Input: part model. Units: mm. Frame: model coordinates. Give positions to 0.01 mm unless a question says otherwise; leave off trailing zeros. Loops run counter-clockwise (first coordinate to the right, second up) from the corner with the lowest first, then second, coordinate; pieces in that order, holes last.
from build123d import *

# Parameters (mm, degrees)
SKETCH1_W          = 600
SKETCH1_H          = 600
PLATE_DEPTH        = 20
SKETCH2_R          = 87.5
BEARING_HOLE_DEPTH = 18
SKETCH3_R          = 84.25
CUT_EXTRUDE2_DEPTH = 18
SKETCH4_W          = 555
SKETCH4_H          = 555
SKETCH4_W_2        = 550
SKETCH4_H_2        = 550
CUT_EXTRUDE3_DEPTH = 10


with BuildPart() as part:
    # Sketch1 → plate (new body)
    with BuildSketch(Plane(origin=(0, 0, 0), x_dir=(1, 0, 0), z_dir=(0, 1, 0))):
        Rectangle(SKETCH1_W, SKETCH1_H)
    extrude(amount=PLATE_DEPTH)

    # Sketch2 → bearing-hole (cut)
    with BuildSketch(Plane(origin=(0, 20, 0), x_dir=(1, 0, 0), z_dir=(0, 1, 0))):
        with Locations(Location((0, 0, 0), (0, 0, 270))):
            Circle(SKETCH2_R)
    extrude(amount=-BEARING_HOLE_DEPTH, mode=Mode.SUBTRACT)

    # Sketch3 → Cut-Extrude2 (cut)
    with BuildSketch(Plane(origin=(0, 2, 0), x_dir=(1, 0, 0), z_dir=(0, 1, 0))):
        with Locations(Location((0, 0, 0), (0, 0, 270))):
            Circle(SKETCH3_R)
    extrude(amount=-CUT_EXTRUDE2_DEPTH, mode=Mode.SUBTRACT)

    # Sketch4 → Cut-Extrude3 (cut)
    with BuildSketch(Plane(origin=(0, 20, 0), x_dir=(1, 0, 0), z_dir=(0, 1, 0))):
        Rectangle(SKETCH4_W, SKETCH4_H)
        Rectangle(SKETCH4_W_2, SKETCH4_H_2, mode=Mode.SUBTRACT)
    extrude(amount=-CUT_EXTRUDE3_DEPTH, mode=Mode.SUBTRACT)


solid = part.part
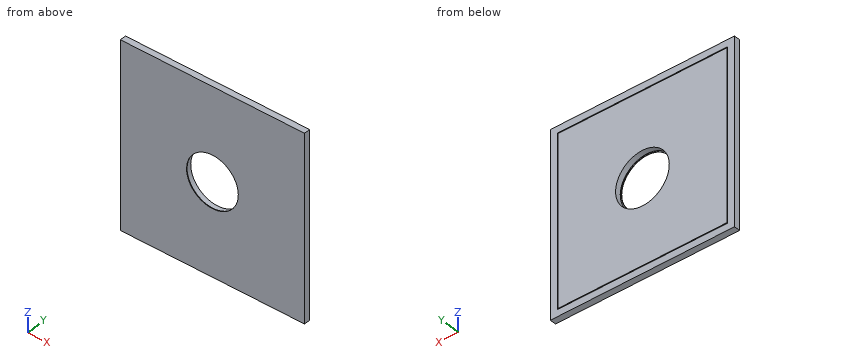
(1) Pin query (flat end, axial travel): pin 1 Ø4 at (x, z) = (191, 232) entering from -Y. Return the tip coordinate at first contact, or that it passes through.
Values follow:
pin 1: stops at y = 0
(2) Cut plane A-A (x = 0). Return the cut outline in (y, z), and give its area (3 significant figures).
Values follow:
outline: (0, -300) - (20, -300) - (20, -277.5) - (10, -277.5) - (10, -275) - (20, -275) - (20, -87.5) - (2, -87.5) - (2, -84.25) - (0, -84.25) - close; (0, 84.25) - (2, 84.25) - (2, 87.5) - (20, 87.5) - (20, 275) - (10, 275) - (10, 277.5) - (20, 277.5) - (20, 300) - (0, 300) - close
area: 8,460 mm2
(3) Cut plane B-B (z = 0). Return the cut outline in (x, y).
Values follow:
outline: (-300, 0) - (-84.25, 0) - (-84.25, 2) - (-87.5, 2) - (-87.5, 20) - (-275, 20) - (-275, 10) - (-277.5, 10) - (-277.5, 20) - (-300, 20) - close; (84.25, 0) - (300, 0) - (300, 20) - (277.5, 20) - (277.5, 10) - (275, 10) - (275, 20) - (87.5, 20) - (87.5, 2) - (84.25, 2) - close
(4) Cut plane C-C (y = 5.75). Return the cut outline in (x, z), and give its area (3 significant figures).
Values follow:
outline: (-300, -300) - (300, -300) - (300, 300) - (-300, 300) - close; hole circle Ø175 at (0, 0)
area: 336,000 mm2
(5) Ray query, probe 1 along X at (y, z) = (16.25, 0); probe 2 along X at (y, z) = (16, -167.5); probe 3 along X at (y, z) = (0.8, 0). Return the intervals inside material, ascending.
Values follow:
probe 1: x = -300 to -277.5, -275 to -87.5, 87.5 to 275, 277.5 to 300
probe 2: x = -300 to -277.5, -275 to 275, 277.5 to 300
probe 3: x = -300 to -84.25, 84.25 to 300
